```python
from build123d import *

# Parameters (mm, degrees)
RAIL_DEPTH      = 230
LPATTERN1_COUNT = 6
LPATTERN1_PITCH = 40


with BuildPart() as part:
    # Sketch2 → Rail (new body)
    with BuildSketch(Plane.XY):
        Polygon((-7.5, 0), (7.5, 0), (7.5, 4.689061216), (5.357142857, 6.333333333), (7.5, 7.97760545), (7.5, 9.5), (-7.5, 9.5), (-7.5, 7.97760545), (-5.357142857, 6.333333333), (-7.5, 4.689061216), align=None)
    extrude(amount=-RAIL_DEPTH)

    # Sketch6 → C'Bore (revolve, cut)
    with BuildSketch(Plane(origin=(0, 0, 0), x_dir=(0, 0, -1), z_dir=(1, 0, 0)), mode=Mode.PRIVATE) as c_bore_sk:
        Polygon((215, 9.5), (218, 9.5), (218, 5), (216.75, 5), (216.75, 0), (215, 0), align=None)
    c_bore = revolve(c_bore_sk.sketch.rotate(Axis((0, 8.904905435, -215), (0, -1, 0)), 180), axis=Axis((0, 8.904905435, -215), (0, -1, 0)), mode=Mode.SUBTRACT)

    # LPattern1: C'Bore ×6
    with Locations(*[(0, 0, i * LPATTERN1_PITCH) for i in range(1, LPATTERN1_COUNT)]):
        add(c_bore, mode=Mode.SUBTRACT)


solid = part.part
```
Can you work these out from the model? Positions are in its coordinate system, mm. A direction names the side the tool comes from. Give positions to 0.01 mm unless a question says otherwise; leave off trailing zeros. Write each loop counter-clockwise with the first axis right and the second up, starting at its lowest first coordinate (ties: lowest second). Pieces come first, ordered by that corner, then holes. Notation, with made-up numbers: (71.5, 62) - (116.5, 62) arc R16 cw to (116.5, 92) - close; hole circle Ø8 at (2, 85). An arc over 180 degrees is marked (long way). Write item = value, one per line. Start each with the question number.
1. On a 3-axis mill with a long thin cutter (end or side, diameter ignored), from which of +Z, -Z, +X, -X, +Y, -Y can I reach the whole of each face in a straight line? I mean faces 1 (the face through (1.8, 7.2, -17.4)), 2 (the face through (0, 5, -230)). Say none if no direction works.
2. Thinking about a two-plate mould opening in X: for faces 3 (the face through (0, 5, 0)), 4 (the face through (7.5, 2, -113)), 5 (the face through (-0.526, 2.465, -13.331)), 6 (the face through (-7.5, 2, -113)), which applies, released by +X, released by -X, zero draft, split by the parting line, or undercut?
3. Imagine slicing it at A-A (z = -157.5). Please give me the cut outline in (x, y), and give its area (3 significant figures).
4. For pin 1 (5 mm diameter, centred on x = 0, z = -15, fed in from +Y); pin 2 (3 mm diameter, centred on x = 0, z = -135, fed in from +Y); pin 3 (1.5 mm diameter, centred on y = 5.5, z = -160, fed in from +X), each with a flat end and sliding along its axis, tell me the tip position at first contact or that it passes through.
5. Imagine slicing it at B-B (y = 3). Please give me the cut outline in (x, z), and give its area (3 significant figures).
6. Please list where these lines run through material, in increasing order: line 1 (X direction, y = 2, z = -215); line 2 (Y direction, x = -2.75, z = -134); line 3 (Y direction, x = 5.75, z = -116).
Worked answers:
q1.face_1 = +Y
q1.face_2 = -Z, +X, -X, +Y, -Y
q2.face_3 = zero draft
q2.face_4 = released by +X
q2.face_5 = undercut
q2.face_6 = released by -X
q3.outline = (-7.5, 0) - (7.5, 0) - (7.5, 4.69) - (5.36, 6.33) - (7.5, 7.98) - (7.5, 9.5) - (-7.5, 9.5) - (-7.5, 7.98) - (-5.36, 6.33) - (-7.5, 4.69) - close
q3.area = 135 mm2
q4.pin_1 = 5
q4.pin_2 = through
q4.pin_3 = 7.42
q5.outline = (-7.5, -230) - (7.5, -230) - (7.5, 0) - (-7.5, 0) - close; hole circle Ø3.5 at (0, -215); hole circle Ø3.5 at (0, -175); hole circle Ø3.5 at (0, -135); hole circle Ø3.5 at (0, -95); hole circle Ø3.5 at (0, -55); hole circle Ø3.5 at (0, -15)
q5.area = 3,390 mm2
q6.line_1 = -7.5 to -1.75, 1.75 to 7.5
q6.line_2 = 0 to 5
q6.line_3 = 0 to 6.03, 6.63 to 9.5
